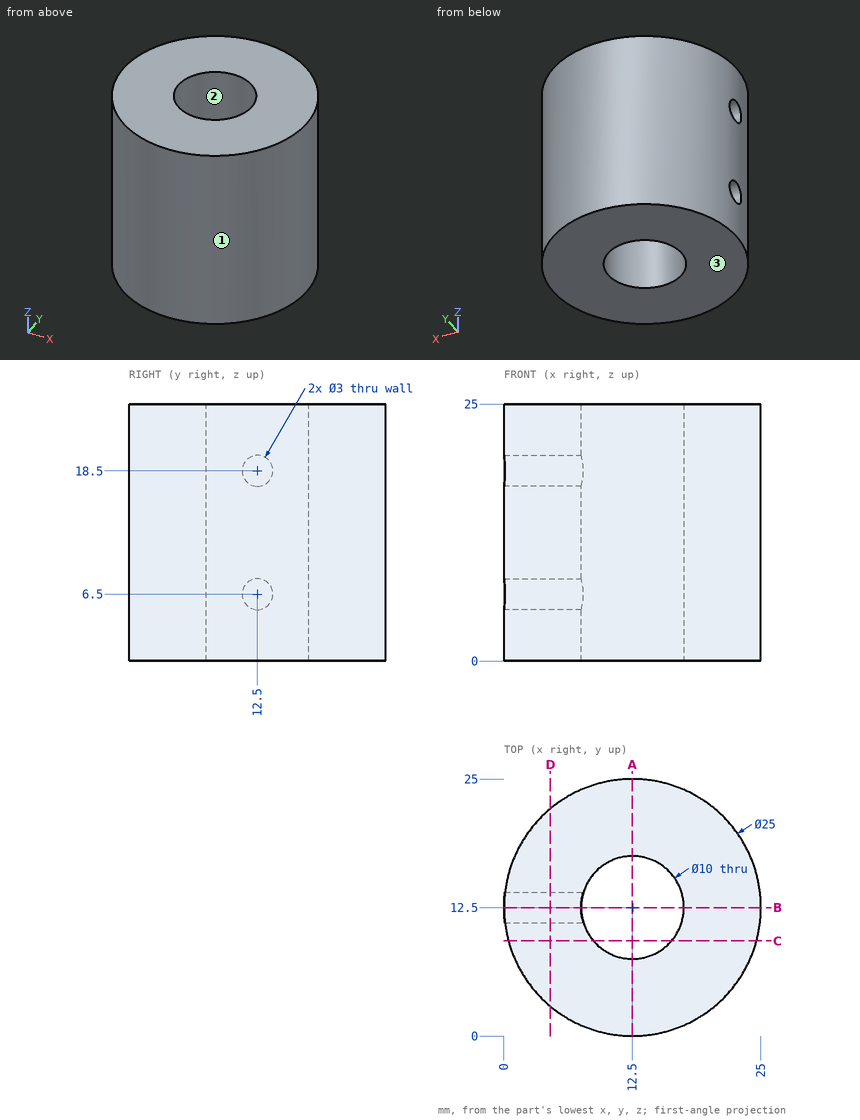
Design review of the part shown in the three views and the two pictorial views. Dimensions are in mm from the part's minimum x, y and z. Round coordinates to 2 decimals unless told otherwise and drop trailing zeros. Write each loop counter-clockwise with the first axis right and the second up, starting at its lowest first coordinate (ties: lowest second). Pieces come first, ordered by that corner, then holes. Notation, with made-up numbers: (63, 80) -> (114, 80) arc R18 cw to (114, 89) -> close; hole circle Ø4 at (13, 8). An arc over 180 degrees is marked (long way). One line per question, with ' | ' between items. Start each with the question number.
1) Add section C-C (y = 9.25). Write out the cut boundary in (x, z).
2) For pin 1 Ø5 at (x, z) = (17.5, 14) entering from -Y; pin 2 Ø8 at (x, z) = (11, 8.5) entering from +Y; pin 3 Ø8 at (y, z) = (21, 21.5) entering from -X; pin 4 Ø6 at (x, z) = (4, 7.5) entering from +Y (3 decimals), all flat-tipped, find the tip position at first contact; note any pin that passes through.
3) Mouldability with a two-part tool opening along Y and no side actions: class the marked faces 1, 2 and 3 as +Y half, -Y half, draft (parallel to the pull), parting line (faces both ways), or undercut.
4) Add section B-B (y = 12.5). Write out the cut boundary in (x, z), and give its area (3 significant figures).
5) Add section D-D (x = 4.5). Write out the cut boundary in (y, z).
6) Add section A-A (x = 12.5). Write out the cut boundary in (y, z).
7) Wall thickness on line 1 along Y through (x, z) = (15.75, 17); line 2 along X through (y, z) = (9.5, 12.5); line 3 along Y through (x, z) = (2.75, 6.5): over which ranges is each line inside the solid? List them lowest first.
Reported:
1) outline: (0.43, 0) -> (8.7, 0) -> (8.7, 25) -> (0.43, 25) -> close; (16.3, 0) -> (24.57, 0) -> (24.57, 25) -> (16.3, 25) -> close
2) pin 1: stops at y = 0.25 | pin 2: stops at y = 25 | pin 3: stops at x = 0.84 | pin 4: stops at y = 23.725
3) face 1: parting line | face 2: undercut | face 3: draft
4) outline: (0, 0) -> (7.5, 0) -> (7.5, 5) -> (0, 5) -> close; (0, 8) -> (7.5, 8) -> (7.5, 17) -> (0, 17) -> close; (0, 20) -> (7.5, 20) -> (7.5, 25) -> (0, 25) -> close; (17.5, 0) -> (25, 0) -> (25, 25) -> (17.5, 25) -> close | area: 330 mm²
5) outline: (2.9, 0) -> (22.1, 0) -> (22.1, 25) -> (2.9, 25) -> close; hole circle Ø3 at (12.5, 6.5); hole circle Ø3 at (12.5, 18.5)
6) outline: (0, 0) -> (7.5, 0) -> (7.5, 25) -> (0, 25) -> close; (17.5, 0) -> (25, 0) -> (25, 25) -> (17.5, 25) -> close
7) line 1: y = 0.43 to 8.7, 16.3 to 24.57 | line 2: x = 0.37 to 8.5, 16.5 to 24.63 | line 3: y = 4.68 to 11, 14 to 20.32
